Geometry check sheet. Reference: the model listing, model coordinates, mm. Round coordinates to 2 decimals unless told otherwise and drop trailing zeros. Write each loop counter-clockwise with the first axis right and the second up, starting at its lowest first coordinate (ties: lowest second). Pieces come first, ordered by that corner, then holes. Notation, with made-up numbers: M 14.5,3.5 L 46.5,3.5 A20 ccw 46.5,11.5 Z; hole C -32,-17.5 d9. An arc over 180 degrees is marked long. Use a Markdown table: item, result.
```python
from build123d import *

# Parameters (mm, degrees)
F1_DEPTH = 25.4
F2_R     = 5.08
F3_R     = 5.08
F4_R     = 12.7
F5_DEPTH = 25.401
F6_R     = 5.08


with BuildPart() as f1:
    # F0 (on Top) → F1 (new body)
    with BuildSketch(Plane.XY):
        Polygon((23.816695, -13.750575), (23.816695, 13.750575), (0, 27.501151), (-23.816695, 13.750575), (-23.816695, -13.750575), (0, -27.501151), align=None)
    extrude(amount=F1_DEPTH)

    # F2
    f2_edges = [f1.edges().sort_by_distance(p)[0] for p in [
        (23.816695, 13.750575, 12.7),
        (0, 27.501151, 12.7),
        (23.816695, -13.750575, 12.7),
        (0, -27.501151, 12.7),
        (-23.816695, -13.750575, 12.7),
        (-23.816695, 13.750575, 12.7),
    ]]
    fillet(f2_edges, radius=F2_R)

    # F3
    f3_edges = [f1.edges().sort_by_distance(p)[0] for p in [
        (11.908348, -20.625863, 25.4),
        (0, -26.715272, 25.4),
        (23.136104, -13.357636, 25.4),
        (-11.908348, -20.625863, 25.4),
        (23.816695, 0, 25.4),
        (-23.136104, -13.357636, 25.4),
        (23.136104, 13.357636, 25.4),
        (-23.816695, 0, 25.4),
        (11.908348, 20.625863, 25.4),
        (-23.136104, 13.357636, 25.4),
        (0, 26.715272, 25.4),
        (-11.908348, 20.625863, 25.4),
        (11.908348, -20.625863, 0),
        (0, -26.715272, 0),
        (23.136104, -13.357636, 0),
        (-11.908348, -20.625863, 0),
        (23.816695, 0, 0),
        (-23.136104, -13.357636, 0),
        (23.136104, 13.357636, 0),
        (-23.816695, 0, 0),
        (11.908348, 20.625863, 0),
        (-23.136104, 13.357636, 0),
        (0, 26.715272, 0),
        (-11.908348, 20.625863, 0),
    ]]
    fillet(f3_edges, radius=F3_R)

    # F4 (on face) → F5 (cut, through all)
    with BuildSketch(Plane.XY.offset(25.4)):
        Circle(F4_R)
    extrude(amount=-F5_DEPTH, mode=Mode.SUBTRACT)

    # F6
    f6_edges = [f1.edges().sort_by_distance(p)[0] for p in [
        (-12.7, 0, 25.4),
        (12.7, 0, 12.7),
        (-12.7, 0, 0),
    ]]
    fillet(f6_edges, radius=F6_R)


solid = f1.part
```
Item 1: Cross-section at A-A, the plane y = 0. Record the cut outline in (x, z), and give its area (3 significant figures).
Outcome:
| item | result |
|---|---|
| outline | M -23.82,5.08 A5.08 ccw -18.74,0 L -17.78,0 A5.08 ccw -12.7,5.08 L -12.7,20.32 A5.08 ccw -17.78,25.4 L -18.74,25.4 A5.08 ccw -23.82,20.32 Z; M 12.7,5.08 A5.08 ccw 17.78,0 L 18.74,0 A5.08 ccw 23.82,5.08 L 23.82,20.32 A5.08 ccw 18.74,25.4 L 17.78,25.4 A5.08 ccw 12.7,20.32 Z |
| area | 520 mm2 |
Item 2: Go/stop test with flat-tipped pins: pin 1 (5 mm diameter, centred on x = -14, z = 3.5, fed in from -Y); pin 2 (12 mm diameter, centred on x = 7.5, z = 10.5, fed in from +Y); pin 3 (1.5 mm diameter, centred on y = -12.5, z = 6, fed in from -X); pin 4 (10 mm diameter, centred on x = -3, y = -7, fed in from +Z). Record where each tip stops, or that it passes through.
Outcome:
| item | result |
|---|---|
| pin 1 | stops at y = -20.72 |
| pin 2 | stops at y = 26.49 |
| pin 3 | stops at x = -23.73 |
| pin 4 | passes through |
Item 3: Cross-section at B-B, the plane z = 14.5. Record the cut outline in (x, y), and give its area (3 significant figures).
Outcome:
| item | result |
|---|---|
| outline | M -23.82,-10.82 A5.08 ccw -21.28,-15.22 L -2.54,-26.03 A5.08 ccw 2.54,-26.03 L 21.28,-15.22 A5.08 ccw 23.82,-10.82 L 23.82,10.82 A5.08 ccw 21.28,15.22 L 2.54,26.03 A5.08 ccw -2.54,26.03 L -21.28,15.22 A5.08 ccw -23.82,10.82 Z; hole C 0,0 d25.4 |
| area | 1,450 mm2 |
Item 4: Mould release check, pull along Y, two halves, no side actions. Record for faces 1 (the face through (-2.75, -12.4, 12.81)), 2 (the face through (-12.04, -20.55, 12.59)), 3 (the face through (-11.276, 19.227, 23.951)), 4 (the face through (-22.29, -0.15, 23.95)): +Y half, -Y half, draft (parallel to the pull), parting line (faces both ways), or undercut.
Outcome:
| item | result |
|---|---|
| face 1 | undercut |
| face 2 | -Y half |
| face 3 | +Y half |
| face 4 | draft |
Item 5: Material ranges on line 1 along Y through (x, z) = (0, 12); line 2 along X through (y, z) = (0.5, 8); line 3 along Y through (x, z) = (3.5, 20), recorded low to high. Write a range as from..to.
Outcome:
| item | result |
|---|---|
| line 1 | y = -26.72..-12.7, 12.7..26.72 |
| line 2 | x = -23.82..-12.69, 12.69..23.82 |
| line 3 | y = -25.48..-12.21, 12.21..25.48 |
